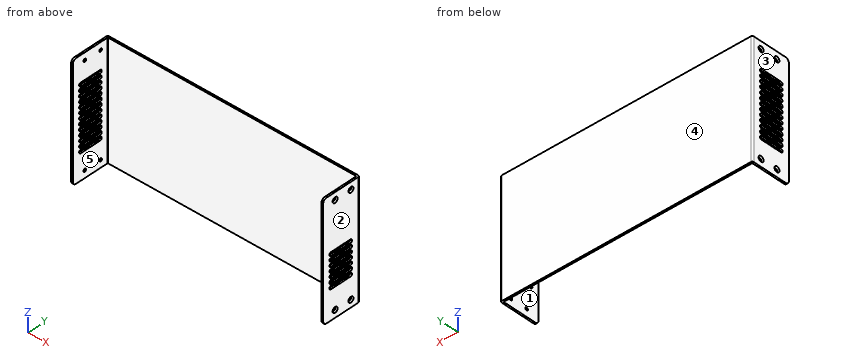
from build123d import *

# Parameters (mm, degrees)
BOSS_EXTRUDE1_DEPTH                             = 135
CSK_FOR_M3_FLAT_HEAD_MACHINE_SCREW1_D           = 3.4
CSK_FOR_M3_FLAT_HEAD_MACHINE_SCREW1_DEPTH       = 5
CSK_FOR_M3_FLAT_HEAD_MACHINE_SCREW1_CSINK_D     = 6.3
CSK_FOR_M3_FLAT_HEAD_MACHINE_SCREW1_CSINK_ANGLE = 90
CSK_FOR_M3_FLAT_HEAD_MACHINE_SCREW1_TIP         = 1.021463052
CSK_FOR_M3_FLAT_HEAD_MACHINE_SCREW2_D           = 3.4
CSK_FOR_M3_FLAT_HEAD_MACHINE_SCREW2_DEPTH       = 5
CSK_FOR_M3_FLAT_HEAD_MACHINE_SCREW2_CSINK_D     = 6.3
CSK_FOR_M3_FLAT_HEAD_MACHINE_SCREW2_CSINK_ANGLE = 90
CSK_FOR_M3_FLAT_HEAD_MACHINE_SCREW2_TIP         = 1.021463052
FILLET1_R                                       = 4
CUT_EXTRUDE1_DEPTH                              = 10
LPATTERN1_COUNT                                 = 13
LPATTERN1_PITCH                                 = 6
CUT_EXTRUDE2_DEPTH                              = 10
LPATTERN2_COUNT                                 = 7
LPATTERN2_PITCH                                 = 6


with BuildPart() as part:
    # Sketch1 → Boss-Extrude1 (new body)
    with BuildSketch(Plane.XY):
        with BuildLine():
            Line((0, 0), (-2, 0))
            Line((-2, 0), (-2, 44.2))
            ThreePointArc((-2, 44.2), (-1.472792206, 45.472792206), (-0.2, 46))
            Line((-0.2, 46), (290.6, 46))
            ThreePointArc((290.6, 46), (291.872792206, 45.472792206), (292.4, 44.2))
            Line((292.4, 44.2), (292.4, 0))
            Line((292.4, 0), (290.4, 0))
            Line((290.4, 0), (290.4, 43.5))
            ThreePointArc((290.4, 43.5), (290.253553391, 43.853553391), (289.9, 44))
            Line((289.9, 44), (0.5, 44))
            ThreePointArc((0.5, 44), (0.146446609, 43.853553391), (0, 43.5))
            Line((0, 43.5), (0, 0))
        make_face()
    extrude(amount=BOSS_EXTRUDE1_DEPTH)

    # CSK for M3 Flat Head Machine Screw1
    with Locations(Plane.ZY.offset(2)):
        with Locations((8.5, 35), (8.5, 15), (126.5, 35), (126.5, 15)):
            CounterSinkHole(CSK_FOR_M3_FLAT_HEAD_MACHINE_SCREW1_D / 2, CSK_FOR_M3_FLAT_HEAD_MACHINE_SCREW1_CSINK_D / 2, depth=CSK_FOR_M3_FLAT_HEAD_MACHINE_SCREW1_DEPTH, counter_sink_angle=CSK_FOR_M3_FLAT_HEAD_MACHINE_SCREW1_CSINK_ANGLE)
            with Locations((0, 0, -(CSK_FOR_M3_FLAT_HEAD_MACHINE_SCREW1_DEPTH + CSK_FOR_M3_FLAT_HEAD_MACHINE_SCREW1_TIP / 2))):  # 118° drill point
                Cone(0, CSK_FOR_M3_FLAT_HEAD_MACHINE_SCREW1_D / 2, CSK_FOR_M3_FLAT_HEAD_MACHINE_SCREW1_TIP, mode=Mode.SUBTRACT)

    # CSK for M3 Flat Head Machine Screw2
    with Locations(Plane(origin=(292.4, 0, 0), x_dir=(0, 0, -1), z_dir=(1, 0, 0))):
        with Locations((-126.5, 35), (-126.5, 15), (-8.5, 35), (-8.5, 15)):
            CounterSinkHole(CSK_FOR_M3_FLAT_HEAD_MACHINE_SCREW2_D / 2, CSK_FOR_M3_FLAT_HEAD_MACHINE_SCREW2_CSINK_D / 2, depth=CSK_FOR_M3_FLAT_HEAD_MACHINE_SCREW2_DEPTH, counter_sink_angle=CSK_FOR_M3_FLAT_HEAD_MACHINE_SCREW2_CSINK_ANGLE)
            with Locations((0, 0, -(CSK_FOR_M3_FLAT_HEAD_MACHINE_SCREW2_DEPTH + CSK_FOR_M3_FLAT_HEAD_MACHINE_SCREW2_TIP / 2))):  # 118° drill point
                Cone(0, CSK_FOR_M3_FLAT_HEAD_MACHINE_SCREW2_D / 2, CSK_FOR_M3_FLAT_HEAD_MACHINE_SCREW2_TIP, mode=Mode.SUBTRACT)

    # Fillet1
    fillet1_edges = [part.edges().sort_by_distance(p)[0] for p in [
        (-1, 0, 0),
        (291.4, 0, 0),
        (291.4, 0, 135),
        (-1, 0, 135),
    ]]
    fillet(fillet1_edges, radius=FILLET1_R)

    # Sketch6 → Cut-Extrude1 (cut)
    with BuildSketch(Plane(origin=(-2, 0, 0), x_dir=(0, 0, -1), z_dir=(1, 0, 0))):
        with BuildLine():
            Line((-101.5, 34.375), (-101.5, 9.8))
            ThreePointArc((-101.5, 9.8), (-103.5, 7.8), (-105.5, 9.8))
            Line((-105.5, 9.8), (-105.5, 34.375))
            ThreePointArc((-105.5, 34.375), (-103.5, 36.375), (-101.5, 34.375))
        make_face()
    cut_extrude1 = extrude(amount=CUT_EXTRUDE1_DEPTH, mode=Mode.SUBTRACT)

    # LPattern1: Cut-Extrude1 ×13
    with Locations(*[(0, 0, -i * LPATTERN1_PITCH) for i in range(1, LPATTERN1_COUNT)]):
        add(cut_extrude1, mode=Mode.SUBTRACT)

    # Sketch7 → Cut-Extrude2 (cut)
    with BuildSketch(Plane(origin=(292.4, 0, 0), x_dir=(0, 0, -1), z_dir=(1, 0, 0))):
        with BuildLine():
            Line((-33.5, 34.375), (-33.5, 9.8))
            ThreePointArc((-33.5, 9.8), (-35.5, 7.8), (-37.5, 9.8))
            Line((-37.5, 9.8), (-37.5, 34.375))
            ThreePointArc((-37.5, 34.375), (-35.5, 36.375), (-33.5, 34.375))
        make_face()
    cut_extrude2 = extrude(amount=-CUT_EXTRUDE2_DEPTH, mode=Mode.SUBTRACT)

    # LPattern2: Cut-Extrude2 ×7
    with Locations(*[(0, 0, i * LPATTERN2_PITCH) for i in range(1, LPATTERN2_COUNT)]):
        add(cut_extrude2, mode=Mode.SUBTRACT)


solid = part.part
For this review, take the finished solid that the model builds, in its own axes (mm). Face numbers are marked on the shaded views. A direction names the side the tool comes from. Round coordinates to 2 decimals unless told otherwise and drop trailing zeros. Loops run counter-clockwise (first coordinate to the right, second up) from the corner with the lowest first, then second, coordinate; pieces in that order, holes last. Notation, with made-up numbers: (-27, -28.75) - (19, -28.75) arc R26 ccw to (19, 4.25) - close; hole circle Ø6 at (89, 16). An arc over 180 degrees is marked (long way). Put each result on its own line as item: value. Start each with the question number.
1. Consider section A-A on x = 234. State the section outline as (y, z) points, plus the area to 3 significant figures.
2. Mouldability with a two-part tool opening along X and no side actions: class the marked faces 3, 4 and 5 as +X half, -X half, draft (parallel to the pull), parting line (faces both ways), or undercut.
3. For probe 1 along Y at (x, z) = (290.65, 8.5); probe 2 along X at (y, z) = (21.5, 16.5); probe 3 along Y at (x, z) = (138, 45.5), list the stretches that pass through material, from the lowest coordinate up. Write a range as [from, to].
4. For the marked faces 1 and 2, list the 3-axis set-ups (+Z, -Z, +X, -X, +Y, -Y) from which the entire face can be reached by the end or side of a thin tool; tool diameter is ignored.
5. Insertion check: P1, Ø4, axis at y = 35, z = 8.5, coming from the +X side. The pin has a flat end and moves straight along its axis. Give the tip position at first contact, or say it passes through.
Result sheet:
1. outline: (44, 0) - (46, 0) - (46, 135) - (44, 135) - close
1. area: 270 mm^2
2. face 3: -X half
2. face 4: draft
2. face 5: undercut
3. probe 1: [0, 13.3], [16.7, 33.3], [36.7, 46]
3. probe 2: [-2, 0], [290.4, 292.4]
3. probe 3: [44, 46]
4. face 1: +Z, -Z, -Y
4. face 2: +Z, -Z, +X, +Y, -Y
5. P1: x = 291.25
